Geometry: final body of the model. Coordinates: model frame, mm. A direction names the side the tool comes from. Give positions to 0.01 mm unless a question says otherwise; leave off trailing zeros. Write each loop counter-clockwise with the first axis right and the second up, starting at its lowest first coordinate (ties: lowest second). Pieces come first, ordered by that corner, then holes. Notation, with made-up numbers: M 10,61 L 67,61 A17 cw 67,93 Z; hole C 21.5,58.5 d9. An arc over 180 degrees is marked long. Use a Markdown table: item, result. Add a question column.
1) Section C-C on y = 12. Return the cut outline in (x, z).
2) Draft query along Z for faces 4 (the flat face through (0, 0, 0)), 5 (the flat face through (0, 8, -27)), 6 (the flat face through (18, 12, 7.752)). Return one class per face: +Z half, -Z half, draft (parallel to the pull), parting line (faces both ways), or undercut.
3) Set-up query: faces 1 (the flat face through (18, 13.689, -15)), 2 (the flat face through (-15, 6, 25)), 3 (the flat face through (0, 17, 0)). Return all of +Z, -Z, +X, -X, +Y, -Y with unobstructed straight access to the full face (end or side cutting, diameter ignored); none if empty.
4) Pin query (flat end, axial travel): pin 1 (6 mm diameter, centred on x = 11.5, z = 7, fed in from -Y); pin 2 (2 mm diameter, centred on y = 5, z = 18.5, fed in from +X). Return the tip coordinate at first contact, or that it passes through.
5) Section A-A on z = -12. Return the cut outline in (x, y), then the cut area to 3 significant figures.
6) Section D-D on z = 19.5. Return the cut outline in (x, y), then the cut area to 3 significant figures.
7) Line query: line 1 (Y direction, x = 18, z = 21.5); line 2 (X direction, y = 9.75, z = -22); line 3 (X direction, y = 5.25, z = 23.5). Output: solid intervals per line, ascending.
8) Section B-B on x = -10.5. Return the cut outline in (y, z), then the cut area to 3 significant figures.
```python
from build123d import *

# Parameters (mm, degrees)
SKETCH1_W           = 40
SKETCH1_H           = 54
BOSS_EXTRUDE1_DEPTH = 17
SKETCH2_W           = 30
SKETCH2_H           = 8
SKETCH2_R           = 0.426133687
CUT_EXTRUDE1_DEPTH  = 5
SKETCH3_W           = 12.848601187
SKETCH3_H           = 4.200504235
SKETCH3_W_2         = 13.095689671
SKETCH3_W_3         = 15.195941788
SKETCH3_H_2         = 4.447592718
SKETCH3_W_4         = 13.095689672
SKETCH3_H_3         = 4.076959992
CUT_EXTRUDE2_DEPTH  = 4


with BuildPart() as part:
    # Sketch1 → Boss-Extrude1 (new body)
    with BuildSketch(Plane(origin=(0, 0, 0), x_dir=(1, 0, 0), z_dir=(0, 1, 0))):
        Rectangle(SKETCH1_W, SKETCH1_H)
    extrude(amount=BOSS_EXTRUDE1_DEPTH)

    # Sketch2 → Cut-Extrude1 (cut)
    with BuildSketch(Plane.XY.offset(27)):
        with Locations((0, 6)):
            Rectangle(SKETCH2_W, SKETCH2_H)
        with Locations((-12.339715026, 8.094368166)):
            Circle(SKETCH2_R, mode=Mode.SUBTRACT)
        with Locations((-9.339715026, 8.094368166)):
            Circle(SKETCH2_R, mode=Mode.SUBTRACT)
        with Locations((-6.339715026, 8.094368166)):
            Circle(SKETCH2_R, mode=Mode.SUBTRACT)
        with Locations((-3.339715026, 8.094368166)):
            Circle(SKETCH2_R, mode=Mode.SUBTRACT)
        with Locations((-0.339715026, 8.094368166)):
            Circle(SKETCH2_R, mode=Mode.SUBTRACT)
        with Locations((2.660284974, 8.094368166)):
            Circle(SKETCH2_R, mode=Mode.SUBTRACT)
        with Locations((5.660284974, 8.094368166)):
            Circle(SKETCH2_R, mode=Mode.SUBTRACT)
        with Locations((8.660284974, 8.094368166)):
            Circle(SKETCH2_R, mode=Mode.SUBTRACT)
        with Locations((11.660284974, 8.094368166)):
            Circle(SKETCH2_R, mode=Mode.SUBTRACT)
        with Locations((-9.339715026, 4.094368166)):
            Circle(SKETCH2_R, mode=Mode.SUBTRACT)
        with Locations((-6.339715026, 4.094368166)):
            Circle(SKETCH2_R, mode=Mode.SUBTRACT)
        with Locations((-3.339715026, 4.094368166)):
            Circle(SKETCH2_R, mode=Mode.SUBTRACT)
        with Locations((-0.339715026, 4.094368166)):
            Circle(SKETCH2_R, mode=Mode.SUBTRACT)
        with Locations((2.660284974, 4.094368166)):
            Circle(SKETCH2_R, mode=Mode.SUBTRACT)
        with Locations((5.660284974, 4.094368166)):
            Circle(SKETCH2_R, mode=Mode.SUBTRACT)
        with Locations((8.660284974, 4.094368166)):
            Circle(SKETCH2_R, mode=Mode.SUBTRACT)
        with Locations((11.660284974, 4.094368166)):
            Circle(SKETCH2_R, mode=Mode.SUBTRACT)
        with Locations((-12.339715026, 4.094368166)):
            Circle(SKETCH2_R, mode=Mode.SUBTRACT)
    extrude(amount=-CUT_EXTRUDE1_DEPTH, mode=Mode.SUBTRACT)

    # Sketch3 → Cut-Extrude2 (cut)
    with BuildSketch(Plane(origin=(20, 0, 0), x_dir=(0, 0, -1), z_dir=(1, 0, 0))):
        with Locations((-16.585814513, 11.588606055)):
            Rectangle(SKETCH3_W, SKETCH3_H)
        with Locations((-1.204556361, 11.588606055)):
            Rectangle(SKETCH3_W_2, SKETCH3_H)
        with Locations((14.609106638, 11.588606055)):
            Rectangle(SKETCH3_W_3, SKETCH3_H)
        with Locations((-16.585814513, 5.040761219)):
            Rectangle(SKETCH3_W, SKETCH3_H_2)
        with Locations((0, 5.040761219)):
            Rectangle(SKETCH3_W_4, SKETCH3_H_3)
    extrude(amount=-CUT_EXTRUDE2_DEPTH, mode=Mode.SUBTRACT)


solid = part.part
```
Found:
| question | item | result |
|---|---|---|
| 1 | outline | M -20,-27 L 20,-27 L 20,-22.21 L 16,-22.21 L 16,-7.01 L 20,-7.01 L 20,-5.34 L 16,-5.34 L 16,7.75 L 20,7.75 L 20,10.16 L 16,10.16 L 16,23.01 L 20,23.01 L 20,27 L -20,27 Z |
| 2 | face 4 | draft |
| 2 | face 5 | -Z half |
| 2 | face 6 | undercut |
| 3 | face 1 | +X |
| 3 | face 2 | +Z |
| 3 | face 3 | +Z, -Z, +X, -X, +Y |
| 4 | pin 1 | y = 0 |
| 4 | pin 2 | x = 16 |
| 5 | outline | M -20,0 L 20,0 L 20,9.49 L 16,9.49 L 16,13.69 L 20,13.69 L 20,17 L -20,17 Z |
| 5 | area | 663 mm² |
| 6 | outline | M -20,0 L 20,0 L 20,2.82 L 16,2.82 L 16,7.26 L 20,7.26 L 20,9.49 L 16,9.49 L 16,13.69 L 20,13.69 L 20,17 L -20,17 Z |
| 6 | area | 645 mm² |
| 7 | line 1 | 0 to 2.82, 7.26 to 9.49, 13.69 to 17 |
| 7 | line 2 | -20 to 16 |
| 7 | line 3 | -20 to -15, 15 to 20 |
| 8 | outline | M 0,-27 L 17,-27 L 17,27 L 10,27 L 10,22 L 2,22 L 2,27 L 0,27 Z |
| 8 | area | 878 mm² |
